Read the model definition and answer for the solid it produces. Units are mm, in the model's axes. A direction names the side the tool comes from. Give positions to 0.01 mm unless a question says otherwise; leave off trailing zeros. Return JSON: item names as keys, results as strings.
```python
from build123d import *

# Parameters (mm, degrees)
SKETCH_1_R          = 1.5
SKETCH_1_R_2        = 1
EXTRUDE_1_DEPTH     = 2
SKETCH_3_R          = 3
CUT_EXTRUDE_2_DEPTH = 1
CUT_EXTRUDE_3_DEPTH = 2
FILLET_3_R          = 1
CHAMFER_2_SIZE      = 0.5


with BuildPart() as part:
    # 草图1 → 凸台-拉伸1 (new body)
    with BuildSketch(Plane(origin=(0, 0, 0), x_dir=(1, 0, 0), z_dir=(0, 1, 0))):
        Polygon((-45, 26.899531218), (45, 26.899531218), (45, -27.100468782), (15, -27.100468782), (0, -12.100468782), (-15, -27.100468782), (-45, -27.100468782), align=None)
        with Locations(Location((-40, 21.399531218, 0), (0, 0, 270))):
            Circle(SKETCH_1_R, mode=Mode.SUBTRACT)
        with Locations(Location((-40, -21.600468782, 0), (0, 0, 270))):
            Circle(SKETCH_1_R, mode=Mode.SUBTRACT)
        with Locations(Location((40, 21.399531218, 0), (0, 0, 270))):
            Circle(SKETCH_1_R, mode=Mode.SUBTRACT)
        with Locations(Location((40, -21.600468782, 0), (0, 0, 270))):
            Circle(SKETCH_1_R, mode=Mode.SUBTRACT)
        with Locations(Location((-9, -2.100468782, 0), (0, 0, 270))):
            Circle(SKETCH_1_R_2, mode=Mode.SUBTRACT)
        with Locations(Location((9, -2.100468782, 0), (0, 0, 270))):
            Circle(SKETCH_1_R_2, mode=Mode.SUBTRACT)
        with Locations(Location((0, 20.899531218, 0), (0, 0, 270))):
            Circle(SKETCH_1_R, mode=Mode.SUBTRACT)
        with BuildLine():
            Line((-26.5, 13.649531218), (-13.5, 13.649531218))
            ThreePointArc((-13.5, 13.649531218), (-12.25, 12.399531218), (-13.5, 11.149531218))
            Line((-13.5, 11.149531218), (-26.5, 11.149531218))
            ThreePointArc((-26.5, 11.149531218), (-27.75, 12.399531218), (-26.5, 13.649531218))
        make_face(mode=Mode.SUBTRACT)
        with BuildLine():
            Line((-26.5, -11.350468782), (-13.5, -11.350468782))
            ThreePointArc((-13.5, -11.350468782), (-12.25, -12.600468782), (-13.5, -13.850468782))
            Line((-13.5, -13.850468782), (-26.5, -13.850468782))
            ThreePointArc((-26.5, -13.850468782), (-27.75, -12.600468782), (-26.5, -11.350468782))
        make_face(mode=Mode.SUBTRACT)
        with BuildLine():
            Line((13.5, 13.649531218), (26.5, 13.649531218))
            ThreePointArc((26.5, 13.649531218), (27.75, 12.399531218), (26.5, 11.149531218))
            Line((26.5, 11.149531218), (13.5, 11.149531218))
            ThreePointArc((13.5, 11.149531218), (12.25, 12.399531218), (13.5, 13.649531218))
        make_face(mode=Mode.SUBTRACT)
        with BuildLine():
            Line((13.5, -11.350468782), (26.5, -11.350468782))
            ThreePointArc((26.5, -11.350468782), (27.75, -12.600468782), (26.5, -13.850468782))
            Line((26.5, -13.850468782), (13.5, -13.850468782))
            ThreePointArc((13.5, -13.850468782), (12.25, -12.600468782), (13.5, -11.350468782))
        make_face(mode=Mode.SUBTRACT)
    extrude(amount=EXTRUDE_1_DEPTH)

    # 草图3 → 切除-拉伸2 (cut)
    with BuildSketch(Plane(origin=(0, 2, 0), x_dir=(1, 0, 0), z_dir=(0, 1, 0))):
        with Locations(Location((0, 20.899531218, 0), (0, 0, 270))):
            Circle(SKETCH_3_R)
    extrude(amount=-CUT_EXTRUDE_2_DEPTH, mode=Mode.SUBTRACT)

    # 草图2 → 切除-拉伸3 (cut)
    with BuildSketch(Plane(origin=(0, 2, 0), x_dir=(1, 0, 0), z_dir=(0, 1, 0))):
        Polygon((-35.541259455, -22.100468782), (-20.523817595, -22.100468782), (-25.773817595, -16.850468782), align=None)
        Polygon((-16.67612236, -21.70552333), (-22.220805057, -16.160840633), (-11.131439663, -16.160840633), align=None)
        Polygon((-40, -14.747868465), (-20.190884311, -4.100468782), (-40, -4.100468782), align=None)
        Polygon((0, 14.899531218), (-5.519575922, -0.129010379), (5.519575922, -0.129010379), align=None)
        Polygon((-1.745892918, -6.775293888), (-9.25, -14.27940097), (-9.25, -6.775293888), align=None)
        Polygon((-35, 21.899531218), (-6, 21.899531218), (-25.23255814, 16.649531218), align=None)
        Polygon((-29.849319142, -0.100468782), (-35.54355148, 14.240560811), (-16.625597549, -0.100468782), align=None)
        Polygon((-40, 17.334853501), (-40, -0.100468782), (-33.077151446, -0.100468782), align=None)
        Polygon((-19.210594542, 8.149531218), (-8.520261517, 8.149531218), (-10.965913691, 1.899531218), align=None)
        Polygon((9.25, -14.27940097), (9.25, -6.775293888), (1.745892918, -6.775293888), align=None)
        Polygon((22.220805057, -16.160840633), (11.131439663, -16.160840633), (16.67612236, -21.70552333), align=None)
        Polygon((20.523817595, -22.100468782), (25.773817595, -16.850468782), (35.541259455, -22.100468782), align=None)
        Polygon((20.190884311, -4.100468782), (40, -4.100468782), (40, -14.747868465), align=None)
        Polygon((8.520261517, 8.149531218), (10.965913691, 1.899531218), (19.210594542, 8.149531218), align=None)
        Polygon((35.54355148, 14.240560811), (16.625597549, -0.100468782), (29.849319142, -0.100468782), align=None)
        Polygon((40, -0.100468782), (33.077151446, -0.100468782), (40, 17.334853501), align=None)
        Polygon((6, 21.899531218), (25.23255814, 16.649531218), (35, 21.899531218), align=None)
    extrude(amount=-CUT_EXTRUDE_3_DEPTH, mode=Mode.SUBTRACT)

    # 圆角3
    fillet_3_edges = [part.edges().sort_by_distance(p)[0] for p in [
        (-45, 1, -26.899531218),
        (45, 1, -26.899531218),
        (45, 1, 27.100468782),
        (15, 1, 27.100468782),
        (0, 1, 12.100468782),
        (-15, 1, 27.100468782),
        (-45, 1, 27.100468782),
    ]]
    fillet(fillet_3_edges, radius=FILLET_3_R)

    # 倒角2
    chamfer_2_edges = [part.edges().sort_by_distance(p)[0] for p in [
        (-27.75, 0, -12.399531218),
        (-20, 0, -11.149531218),
        (-12.25, 0, -12.399531218),
        (-20, 0, -13.649531218),
        (-27.75, 2, -12.399531218),
        (-20, 2, -11.149531218),
        (-12.25, 2, -12.399531218),
        (-20, 2, -13.649531218),
        (-27.75, 0, 12.600468782),
        (-20, 0, 13.850468782),
        (-12.25, 0, 12.600468782),
        (-20, 0, 11.350468782),
        (-27.75, 2, 12.600468782),
        (-20, 2, 13.850468782),
        (-12.25, 2, 12.600468782),
        (-20, 2, 11.350468782),
        (-9, 0, 1.100468782),
        (-9, 2, 1.100468782),
        (-40, 0, -22.899531218),
        (-40, 2, -22.899531218),
        (-40, 0, 20.100468782),
        (-40, 2, 20.100468782),
        (40, 0, -22.899531218),
        (40, 2, -22.899531218),
        (40, 0, 20.100468782),
        (40, 2, 20.100468782),
        (12.25, 0, -12.399531218),
        (20, 0, -11.149531218),
        (27.75, 0, -12.399531218),
        (20, 0, -13.649531218),
        (12.25, 2, -12.399531218),
        (20, 2, -11.149531218),
        (27.75, 2, -12.399531218),
        (20, 2, -13.649531218),
        (9, 0, 1.100468782),
        (9, 2, 1.100468782),
        (12.25, 0, 12.600468782),
        (20, 0, 13.850468782),
        (27.75, 0, 12.600468782),
        (20, 0, 11.350468782),
        (12.25, 2, 12.600468782),
        (20, 2, 13.850468782),
        (27.75, 2, 12.600468782),
        (20, 2, 11.350468782),
    ]]
    chamfer(chamfer_2_edges, length=CHAMFER_2_SIZE)


solid = part.part
```
Q1. A cutting plane is placed at A-A (z = -6.5). Give the number of separate pieces and of enclosed holes in the cut face, and give its area (3 significant figures).
Values:
{"separate pieces": "8", "enclosed holes": "0", "area": "90.4 mm²"}
Q2. Consider L1, parallel to X at y = 0.1, z = 10.5; L2, parallel to Z at x = -11, y = 0.3; L3, parallel to Z at x = 13, y = 1.65. Determine where each line is inside the solid, lowest interval first.
Values:
{"L1": "x = -45 to -40, -32.1 to -9.25, -5.47 to 5.47, 9.25 to 32.1, 40 to 45", "L2": "z = -26.9 to -21.9, -20.53 to -8.15, -1.93 to 23.1", "L3": "z = -26.9 to -21.9, -19.99 to -13.71, -11.09 to -8.15, -3.44 to 11.29, 13.91 to 16.16, 18.03 to 25.1"}
Q3. For faces 3 (the flat face through (-1.3, 1, -19.6)), 4 (the flat face through (40, 1, 9)), 5 (the conical face through (27.89, 0.36, 12.57)), determine the directions among +Z, -Z, +X, -X, +Y, -Y from which every point of the face is accessible in a straight line to the end or side of a thin tool.
Values:
{"face 3": "+Y", "face 4": "+Y, -Y", "face 5": "-Y"}
Q4. Determine the mould class of faces 1 (the flat face through (32.657, 1.014, -6.97)), 2 (the flat face through (11, 2, 0)) for opening direction X: released by +X, released by -X, zero draft, split by the parting line, or undercut.
Values:
{"face 1": "undercut", "face 2": "zero draft"}
Q5. Given pin 1 (1.8 mm diameter, centred on x = -40, z = -21.4, fed in from +Y); pin 2 (1 mm diameter, centred on x = -5, y = 0.5, fed in from +Z), each flat-ended and moving along its own axis, determine where each tip first touches the part or whether it passes through.
Values:
{"pin 1": "passes through", "pin 2": "stops at z = 17.6"}
